The drawing under review shows one solid part. Ordinate dimensions are in mm from its lowest x, y, z. A direction names the side the tool comes from. Round coordinates to 2 decimals unless told otherwise and drop trailing zeros. Loops run counter-clockwise (first coordinate to the right, second up) from the corner with the lowest first, then second, coordinate; pieces in that order, holes last. Notation, with made-up numbers: (39.5, -37) - (59.5, -37) arc R24 ccw to (59.5, -17) - close; hole circle Ø10 at (52, 8). An arc over 180 degrees is marked (long way). Answer as CSV lines item,"result".
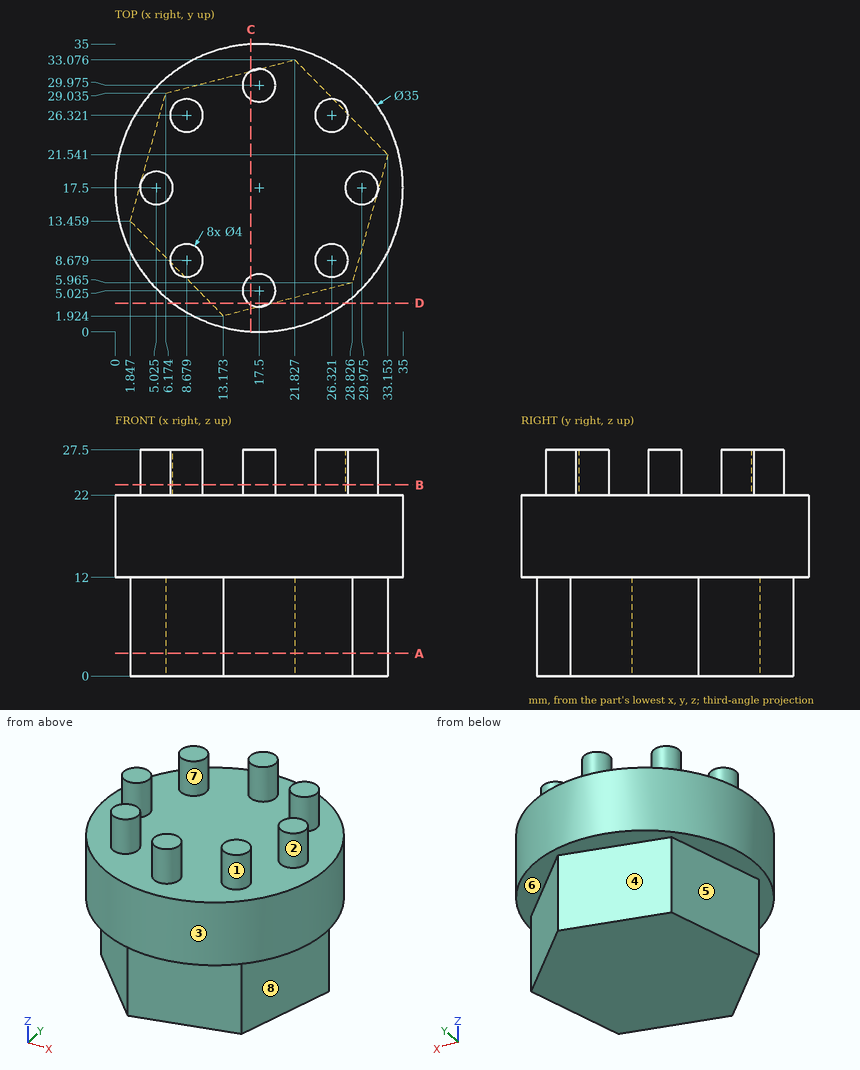
1. Tool access review of the marked faces 5, 6, 7 and 8: name each direction out of +Z, -Z, +X, -X, +Y, -Y from which nothing blocks a thin tool from reaching the whole face with its end or side.
Numbers:
face 5,"-Z, -X, +Y"
face 6,"-Z"
face 7,"+Z"
face 8,"-Z, +X, -Y"
2. Clearance check with flat-ended pins moving along their axes: pin 1 (6 mm diameter, centred on x = 30, y = 14, fed in from -Z); pin 2 (8 mm diameter, centred on y = 8.5, z = 16.5, fed in from +X); pin 3 (8 mm diameter, centred on x = 28, z = 23.5, fed in from -Y); pin 4 (10 mm diameter, centred on y = 9.5, z = 20, fed in from +X). State where each tip first meets the part, or that it passes through.
Numbers:
pin 1,"stops at z = 0"
pin 2,"stops at x = 34.27"
pin 3,"stops at y = 1.37"
pin 4,"stops at x = 34.74"
3. Wall thickness on probe 1 along Z at (x, y) = (20.5, 29); probe 2 along Z at (x, y) = (32, 11.5); probe 3 along X at (y, z) = (17, 26): over which ranges is each line inside the solid? List them lowest first.
Numbers:
probe 1,"z = 0 to 22"
probe 2,"z = 12 to 22"
probe 3,"x = 3.09 to 6.96, 28.04 to 31.91"
4. Take a section at D-D (y = 3.5). State the section outline as (x, z) points (1 decimal), plus the area to 3 significant figures.
Numbers:
outline,"(7, 12) - (11.6, 12) - (11.6, 0) - (19.3, 0) - (19.3, 12) - (28, 12) - (28, 22) - (18.8, 22) - (18.8, 27.5) - (16.2, 27.5) - (16.2, 22) - (7, 22) - close"
area,"316 mm²"
5. Take a section at C-C (x = 16.5). State the section outline as (y, z) points.
Numbers:
outline,"(0.03, 12) - (2.78, 12) - (2.78, 0) - (31.7, 0) - (31.7, 12) - (34.97, 12) - (34.97, 22) - (31.71, 22) - (31.71, 27.5) - (28.24, 27.5) - (28.24, 22) - (6.76, 22) - (6.76, 27.5) - (3.29, 27.5) - (3.29, 22) - (0.03, 22) - close"
6. Take a section at B-B (z = 23.25). State the section outline as (x, y) points (1 decimal).
Numbers:
outline,"circle Ø4 at (5, 17.5); circle Ø4 at (8.7, 8.7); circle Ø4 at (8.7, 26.3); circle Ø4 at (17.5, 5); circle Ø4 at (17.5, 30); circle Ø4 at (26.3, 8.7); circle Ø4 at (26.3, 26.3); circle Ø4 at (30, 17.5)"
7. Take a section at A-A (z = 2.75). State the section outline as (x, y) points (1 decimal).
Numbers:
outline,"(1.8, 13.5) - (13.2, 1.9) - (28.8, 6) - (33.2, 21.5) - (21.8, 33.1) - (6.2, 29) - close"
8. Draft analysis for pull direction X (two halves, no side actions). For the marked faces 1, 2, 3 and 4, state which applies: +X half, -X half, draft (parallel to the pull), parting line (faces both ways), or undercut.
Numbers:
face 1,"undercut"
face 2,"undercut"
face 3,"parting line"
face 4,"-X half"
